from build123d import *

# Parameters (mm, degrees)
F0_W        = 25.4
F0_H        = 25.4
F0_W_2      = 19.05
F0_H_2      = 19.05
F1_DEPTH    = 127
F2_T1_DEPTH = 152.4
F2_T3_DEPTH = 50.8


# Not quite as in the source:
# - a fillet or chamfer that OpenCascade refuses, or shapes differently, is made with other operations: its cross-section is extruded or revolved along the edge and cut away or added


with BuildPart() as f1:
    # F0 (on Front) → F1 (new body)
    with BuildSketch(Plane.XZ):
        Rectangle(F0_W, F0_H)
        Rectangle(F0_W_2, F0_H_2, mode=Mode.SUBTRACT)
    extrude(amount=F1_DEPTH)

    # F2: fillet of radius 5.08 on 8 edges, made by hand

    # F2_s2 → F2_t1 (cut)
    with BuildSketch(Plane.XZ.offset(-12.7)):
        with BuildLine():
            ThreePointArc((12.7, 7.62), (11.2121024484, 11.2121024484), (7.62, 12.7))
            Line((7.62, 12.7), (12.7, 12.7))
            Line((12.7, 12.7), (12.7, 7.62))
        make_face()
        with BuildLine():
            ThreePointArc((-12.7, 7.62), (-11.2121024484, 11.2121024484), (-7.62, 12.7))
            Line((-7.62, 12.7), (-12.7, 12.7))
            Line((-12.7, 12.7), (-12.7, 7.62))
        make_face()
        with BuildLine():
            ThreePointArc((-12.7, -7.62), (-11.2121024484, -11.2121024484), (-7.62, -12.7))
            Line((-7.62, -12.7), (-12.7, -12.7))
            Line((-12.7, -12.7), (-12.7, -7.62))
        make_face()
        with BuildLine():
            ThreePointArc((7.62, -12.7), (11.2121024484, -11.2121024484), (12.7, -7.62))
            Line((12.7, -7.62), (12.7, -12.7))
            Line((12.7, -12.7), (7.62, -12.7))
        make_face()
    extrude(amount=F2_T1_DEPTH, mode=Mode.SUBTRACT)

    # F2_s4 → F2_t3 (cut)
    with BuildSketch(Plane.YZ.offset(-25.4)):
        with BuildLine():
            ThreePointArc((-5.08, 12.7), (-1.4878975516, 11.2121024484), (0, 7.62))
            Line((0, 7.62), (0, 12.7))
            Line((0, 12.7), (-5.08, 12.7))
        make_face()
        with BuildLine():
            ThreePointArc((-121.92, 12.7), (-125.5121024484, 11.2121024484), (-127, 7.62))
            Line((-127, 7.62), (-127, 12.7))
            Line((-127, 12.7), (-121.92, 12.7))
        make_face()
        with BuildLine():
            ThreePointArc((-5.08, -12.7), (-1.4878975516, -11.2121024484), (0, -7.62))
            Line((0, -7.62), (0, -12.7))
            Line((0, -12.7), (-5.08, -12.7))
        make_face()
        with BuildLine():
            ThreePointArc((-121.92, -12.7), (-125.5121024484, -11.2121024484), (-127, -7.62))
            Line((-127, -7.62), (-127, -12.7))
            Line((-127, -12.7), (-121.92, -12.7))
        make_face()
    extrude(amount=F2_T3_DEPTH, mode=Mode.SUBTRACT)


solid = f1.part
Could you check a few things on this model? Use its own coordinates, in mm. A direction names the side the tool comes from. Coordinates: 2 decimals unless noted, no trailing zeros. Order: outer loops, then holes, each group sorted by start corner. A loop starts at its lowest first (then second) coordinate and runs counter-clockwise, first axis right, second up.
Q1. Will this pin go through, and if not, where does the flat tip stop? pin 1 (8 mm diameter, centred on x = 2, z = 7, fed in from +Y).
Q2. Please list where these lines run through material, in increasing order: L1, parallel to X at y = -21, z = 3.25 (3 decimals); L2, parallel to X at y = -57.5, z = 8.5 (3 decimals).
Q3. Suppose I cut it at B-B on x = 5.5. Please give me the cut outline in (y, z) (3 decimals), and give its area (3 significant figures).
Q4. Which directions (+Z, -Z, +X, -X, +Y, -Y) give clear straight access to the entire face, cutting with the end or side of a thin tool? Please do faces 4 (the cylindrical face through (-11.251, -62.611, 11.172)), 5 (the flat face through (0, -63, 9.525)).
Q5. Suppose I cut it at C-C on y = -83. Please give me the cut outline in (x, z) (3 decimals).
Q6. Suppose I cut it at A-A on z = 3.75. Please give me the cut outline in (x, y) (3 decimals).
Q7. Thinking about a two-plate mould opening in Z: for faces 1 (the cylindrical face through (-0.178, -1.528, 11.251)), 2 (the cylindrical face through (11.172, -62.611, -11.251)), 3 (the flat face through (9.525, -63, 0)), which applies, released by +Z, released by -Z, zero draft, split by the parting line, or undercut?
Answer:
1. pin 1: stops at y = -0.37
2. L1: x = -12.7 to -9.525, 9.525 to 12.7
2. L2: x = -12.623 to -9.525, 9.525 to 12.623
3. outline: (-126.629, -9.525) arc R5.08 ccw to (-121.92, -12.7) - (-5.08, -12.7) arc R5.08 ccw to (-0.371, -9.525) - close; (-126.629, 9.525) - (-0.371, 9.525) arc R5.08 ccw to (-5.08, 12.7) - (-121.92, 12.7) arc R5.08 ccw to start
3. area: 785 mm2
4. face 4: +Z, -X, +Y, -Y
4. face 5: +Y, -Y
5. outline: (-12.7, -7.62) arc R5.08 ccw to (-7.62, -12.7) - (7.62, -12.7) arc R5.08 ccw to (12.7, -7.62) - (12.7, 7.62) arc R5.08 ccw to (7.62, 12.7) - (-7.62, 12.7) arc R5.08 ccw to (-12.7, 7.62) - close; hole (-9.525, -9.525) - (9.525, -9.525) - (9.525, 9.525) - (-9.525, 9.525) - close
6. outline: (-12.7, -127) - (-9.525, -127) - (-9.525, 0) - (-12.7, 0) - close; (9.525, -127) - (12.7, -127) - (12.7, 0) - (9.525, 0) - close
7. face 1: released by +Z
7. face 2: released by -Z
7. face 3: undercut
